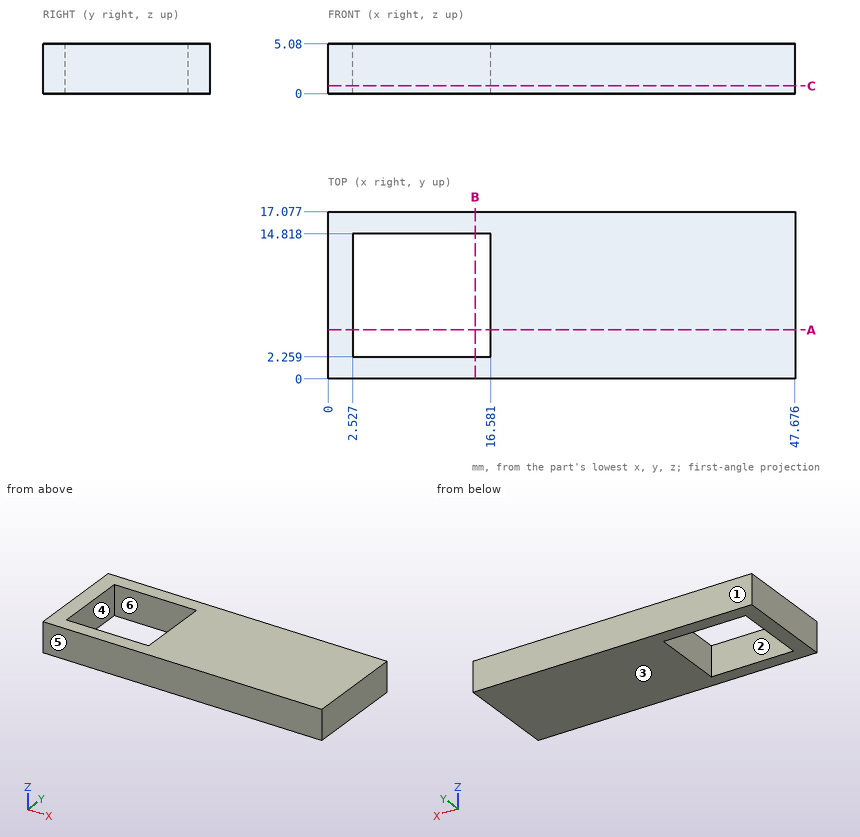
The figure shows three views and two pictorial views of one solid part (mm, origin at its lowest corner). Answer the questions. A direction names the side the tool comes from. Give positions to 0.01 mm unless a question says otherwise; leave off trailing zeros. Order: outer loops, then holes, each group sorted by start corner. A loop starts at its lowest first (then second) coordinate and runs counter-clockwise, first axis right, second up. Notation, with made-up numbers: (51.25, 70.25) -> (72.25, 70.25) arc R22 cw to (72.25, 81.25) -> close; hole circle Ø2 at (82, 13.5). An arc over 180 degrees is marked (long way). Answer as a JSON object with one key per item and string values. Group by question number.
Item 1: The part is cut by section C-C on z = 0.8. Write down the section's boundary in (x, y).
Item 2: Consider L1, parallel to Y at x = 4, z = 0.8; L2, parallel to X at y = 4.5, z = 1.95. Determine where each line is inside the solid, lowest interval first. Write a range as from..to.
Item 3: A tool of negligible diameter and unlimited length cuts with its end or side. For the marked faces 1 and 2, from which of +Z, -Z, +X, -X, +Y, -Y can it reach the whole face along a straight path? Write none if from no direction.
Item 4: Determine the mould class of the marked faces 3, 4, 5 and 6 for opening direction Y: pulls with the +Y half, pulls with the -Y half, needs draft (parallel to the pull), parting line crosses it, or undercut.
Item 5: A flat-ended cylindrical pin translates along its axis: pin 1 (1.5 mm diameter, centred on x = 12, z = 1.5, fed in from -Y). Find the tip coordinate at first contact, or state that the pin passes through.
Item 6: The part is cut by section A-A on y = 5. Write down the section's boundary in (x, z), and give its area (3 significant figures).
Item 7: The part is cut by section B-B on x = 15. Write down the section's boundary in (y, z).
Result set:
{
 "1": {"outline": "(0, 0) -> (47.68, 0) -> (47.68, 17.08) -> (0, 17.08) -> close; hole (2.53, 2.26) -> (16.58, 2.26) -> (16.58, 14.82) -> (2.53, 14.82) -> close"},
 "2": {"L1": "0..2.26, 14.82..17.08", "L2": "0..2.53, 16.58..47.68"},
 "3": {"face 1": "+Z, -Z, +X, -X, +Y", "face 2": "+Z, -Z"},
 "4": {"face 3": "needs draft", "face 4": "undercut", "face 5": "pulls with the -Y half", "face 6": "undercut"},
 "5": {"pin 1": "y = 0"},
 "6": {"outline": "(0, 0) -> (2.53, 0) -> (2.53, 5.08) -> (0, 5.08) -> close; (16.58, 0) -> (47.68, 0) -> (47.68, 5.08) -> (16.58, 5.08) -> close", "area": "171 mm²"},
 "7": {"outline": "(0, 0) -> (2.26, 0) -> (2.26, 5.08) -> (0, 5.08) -> close; (14.82, 0) -> (17.08, 0) -> (17.08, 5.08) -> (14.82, 5.08) -> close"}
}
